Design review of the part built by this model. Coordinates are the model's own, in mm. Face numbers are marked on the shaded views. A direction names the side the tool comes from. Give positions to 0.01 mm unless a question says otherwise; leave off trailing zeros. Write each loop counter-clockwise with the first axis right and the second up, starting at its lowest first coordinate (ties: lowest second). Pieces come first, ordered by that corner, then holes. Notation, with made-up numbers: (35.25, -37) -> (91.25, -37) arc R7 cw to (91.25, -28) -> close; hole circle Ø7 at (-30, 0). An arc over 180 degrees is marked (long way). Write each question's results on one line, items separated by ' | '. Start each with the question number.
(1) Clearance check with flat-ended pins moving along their axes: pin 1 (1.1 mm diameter, centred on x = -34, y = -8, fed in from +Z); pin 2 (5 mm diameter, centred on x = 0.5, z = -31, fed in from +Y); pin 3 (5 mm diameter, centred on y = -5, z = -13.5, fed in from -X); pin 4 (2.5 mm diameter, centred on x = -0.15, y = -4.8, fed in from -Z). State where each tip first meets the part, or that it passes through.
(2) Take a section at B-B (z = -13). State the section outline as (x, y) points.
(3) Take a section at D-D (z = -30). State the section outline as (x, y) points, plus the area to 3 significant figures.
(4) Mouldability with a two-part tool opening along Y and no side actions: class the marked faces 1, 2 and 3 as released by +Y, released by -Y, zero draft, split by the parting line, or undercut.
(5) Take a section at C-C (z = -1.15). State the section outline as (x, y) points.
(6) Take a section at A-A (y = -2.5). State the section outline as (x, z) points, plus the area to 3 significant figures.
(7) To check wall thickness, follow probe 1 along Y at (x, z) = (-5.5, -12); probe 2 along X at (y, z) = (-15.9, -30); probe 3 along Z at (x, y) = (-1.5, 5). State the ranges of each line that lie inside material, in increasing order.
(8) For the marked faces 4, 5 and 6, list the 3-axis set-ups (+Z, -Z, +X, -X, +Y, -Y) from which the entire face can be reached by the end or side of a thin tool; tool diameter is ignored.
from build123d import *

# Parameters (mm, degrees)
ESBO_O3_W                 = 15
ESBO_O3_H                 = 34.8
RESSALTO_EXTRUS_O1_DEPTH  = 3
ESBO_O5_W                 = 15
ESBO_O5_H                 = 3
RESSALTO_EXTRUS_O2_DEPTH  = 18.6
ESBO_O6_W                 = 15
ESBO_O6_H                 = 3
RESSALTO_EXTRUS_O3_DEPTH  = 35
ESBO_O8_R                 = 1.5
CORTE_EXTRUS_O1_DEPTH     = 15
ESBO_O10_R                = 1.5
CORTE_EXTRUS_O3_DEPTH     = 15
CHANFRO2_SIZE             = 1.6
RESSALTO_EXTRUS_O5_DEPTH  = 15
ESBO_O14_R                = 1.5
RESSALTO_EXTRUS_O7_DEPTH  = 3
RESSALTO_EXTRUS_O9_DEPTH  = 26.8
CHANFRO6_SIZE             = 1
CHANFRO7_SIZE             = 1
CHANFRO8_SIZE             = 1
ESBO_O19_W                = 4.68
ESBO_O19_H                = 19.93
ESBO_O19_R                = 1.5
RESSALTO_EXTRUS_O10_DEPTH = 2
ESBO_O17_R                = 1.5
CORTE_EXTRUS_O4_DEPTH     = 7
CHANFRO4_SIZE             = 1
CHANFRO10_SIZE            = 1.6
CHANFRO11_SIZE            = 0.5


with BuildPart() as part:
    # Esboço3 → Ressalto-extrusão1 (new body)
    with BuildSketch(Plane.XY):
        with Locations((-2.101786792, 0.972895567)):
            Rectangle(ESBO_O3_W, ESBO_O3_H)
    extrude(amount=RESSALTO_EXTRUS_O1_DEPTH)

    # Esboço5 → Ressalto-extrusão2 (add)
    with BuildSketch(Plane(origin=(0, 0, 0), x_dir=(-1, 0, 0), z_dir=(0, 0, -1))):
        with Locations((2.101786792, 16.872895567)):
            Rectangle(ESBO_O5_W, ESBO_O5_H)
    extrude(amount=RESSALTO_EXTRUS_O2_DEPTH)

    # Esboço6 → Ressalto-extrusão3 (add)
    with BuildSketch(Plane(origin=(0, 0, 0), x_dir=(-1, 0, 0), z_dir=(0, 0, -1))):
        with Locations((2.101786792, -14.927104433)):
            Rectangle(ESBO_O6_W, ESBO_O6_H)
    extrude(amount=RESSALTO_EXTRUS_O3_DEPTH)

    # Esboço8 → Corte-extrusão1 (cut)
    with BuildSketch(Plane(origin=(0, 0, 0), x_dir=(-1, 0, 0), z_dir=(0, 0, -1))):
        with Locations((0.151786792, 12.802895567)):
            Circle(ESBO_O8_R)
        with Locations((0.151786792, -4.797104433)):
            Circle(ESBO_O8_R)
    extrude(amount=-CORTE_EXTRUS_O1_DEPTH, mode=Mode.SUBTRACT)

    # Esboço10 → Corte-extrusão3 (cut)
    with BuildSketch(Plane(origin=(0, -13.427104433, 0), x_dir=(1, 0, 0), z_dir=(0, 1, 0))):
        with Locations(Location((-2.101786792, 30, 0), (0, 0, 270))):
            Circle(ESBO_O10_R)
    extrude(amount=-CORTE_EXTRUS_O3_DEPTH, mode=Mode.SUBTRACT)

    # Chanfro2
    chanfro2_edges = [part.edges().sort_by_distance(p)[0] for p in [
        (-2.101786792, -13.427104433, -31.5),
    ]]
    chamfer(chanfro2_edges, length=CHANFRO2_SIZE)

    # Esboço11 → Ressalto-extrusão5 (add)
    with BuildSketch(Plane(origin=(5.398213208, 0, 0), x_dir=(0, 0, -1), z_dir=(1, 0, 0))):
        Polygon((7e-08, -7.367104433), (20, -7.367104433), (26.06, -13.427104433), (21.81735926, -13.427104379), (18.757359313, -10.367104433), (3.2e-08, -10.367104433), align=None)
    extrude(amount=-RESSALTO_EXTRUS_O5_DEPTH)

    # Esboço14 → Ressalto-extrusão7 (add)
    with BuildSketch(Plane.XY.offset(-7.35)):
        Polygon((-31.721786792, 6.502895567), (-31.721786792, -7.367104433), (-9.601786792, -7.367104433), (-9.601786792, -16.427104433), (-31.721786792, -16.427104433), (-36.401786792, -16.427104433), (-36.401786792, 6.502895567), align=None)
        with Locations((-34.001786792, 4.002895567)):
            Circle(ESBO_O14_R, mode=Mode.SUBTRACT)
    extrude(amount=RESSALTO_EXTRUS_O7_DEPTH)

    # Esboço16 → Ressalto-extrusão9 (add)
    with BuildSketch(Plane.ZY.offset(9.601786792)):
        Polygon((0, -13.427104433), (-4.35, -13.427104433), (-4.35, -16.427104433), (3, -16.427104433), (3, -13.427104433), align=None)
    extrude(amount=RESSALTO_EXTRUS_O9_DEPTH)

    # Chanfro6
    chanfro6_edges = [part.edges().sort_by_distance(p)[0] for p in [
        (-9.601786792, -11.897104433, -4.35),
        (-9.601786792, -11.897104433, -7.35),
    ]]
    chamfer(chanfro6_edges, length=CHANFRO6_SIZE)

    # Chanfro7
    chanfro7_edges = [part.edges().sort_by_distance(p)[0] for p in [
        (-9.601786792, -13.427104433, -14.58367963),
    ]]
    chamfer(chanfro7_edges, length=CHANFRO7_SIZE)

    # Chanfro8
    chanfro8_edges = [part.edges().sort_by_distance(p)[0] for p in [
        (-9.601786792, -13.427104433, -7.35),
    ]]
    chamfer(chanfro8_edges, length=CHANFRO8_SIZE)

    # Esboço19 → Ressalto-extrusão10 (add)
    with BuildSketch(Plane.XY.offset(-4.35)):
        with Locations((-34.061786792, -3.462104433)):
            Rectangle(ESBO_O19_W, ESBO_O19_H)
        with Locations((-34.001786792, 4.002895567)):
            Circle(ESBO_O19_R, mode=Mode.SUBTRACT)
    extrude(amount=RESSALTO_EXTRUS_O10_DEPTH)

    # Esboço17 → Corte-extrusão4 (cut)
    with BuildSketch(Plane(origin=(0, -13.427104433, 0), x_dir=(1, 0, 0), z_dir=(0, 1, 0))):
        with Locations(Location((-23.001786792, 1.15, 0), (0, 0, 270))):
            Circle(ESBO_O17_R)
    extrude(amount=-CORTE_EXTRUS_O4_DEPTH, mode=Mode.SUBTRACT)

    # Chanfro4
    chanfro4_edges = [part.edges().sort_by_distance(p)[0] for p in [
        (-23.001786792, -13.427104433, 3),
        (-36.401786792, -14.927104433, 3),
        (-2.101786792, 18.372895567, 3),
        (-9.601786792, 2.472895567, 3),
        (5.398213208, 16.872895567, -18.6),
        (-9.601786792, 16.872895567, -18.6),
        (-2.101786792, 18.372895567, -18.6),
        (-36.401786792, -13.427104433, 0.325),
        (5.398213208, -11.897104433, 0),
        (5.398213208, -13.427104433, -30.53),
        (-9.601786792, -13.427104433, -30.53),
        (5.398213208, -14.927104433, -35),
        (-9.601786792, -14.927104433, -35),
        (-2.101786792, -13.427104433, -35),
        (5.398213208, -13.427104433, -10.90867963),
        (-9.601786792, -11.897104433, 0),
        (5.398213208, -10.397104433, -23.03),
        (-9.601786792, -12.397104433, -20.787359313),
        (-9.601786792, -10.367104433, -2.175000016),
        (-9.601786792, -10.397104433, -23.03),
        (5.398213208, -10.367104433, -9.378679672),
        (5.398213208, -11.897104406, -20.287359286),
        (-9.601786792, 18.372895567, -7.8),
        (5.398213208, 18.372895567, -7.8),
        (-9.601786792, -10.367104433, -13.053679656),
        (5.398213208, 0.972895567, 3),
        (-20.661786792, -7.367104433, -4.35),
        (-20.661786792, -7.367104433, -7.35),
        (-31.721786792, 6.502895567, -4.85),
        (-36.401786792, 6.502895567, -4.85),
    ]]
    chamfer(chanfro4_edges, length=CHANFRO4_SIZE - 0.0001)  # a hair under: the kernel refuses the full size

    # Chanfro10
    chanfro10_edges = [part.edges().sort_by_distance(p)[0] for p in [
        (-23.001786792, -13.427104433, -2.65),
    ]]
    chamfer(chanfro10_edges, length=CHANFRO10_SIZE)

    # Chanfro11
    chanfro11_edges = [part.edges().sort_by_distance(p)[0] for p in [
        (-31.721786792, -3.962054433, -2.35),
        (-36.401786792, -5.462054433, -7.35),
        (-36.401786792, -4.462004433, -2.35),
        (-34.061786792, 6.502895567, -7.35),
        (-32.221736792, 6.002945567, -7.35),
        (-35.901836792, 6.002945567, -7.35),
        (-34.061786792, 6.502895567, -2.35),
        (-32.221736792, 6.002945567, -2.35),
        (-35.901836792, 6.002945567, -2.35),
        (-31.721786792, -1.432004433, -7.35),
    ]]
    chamfer(chanfro11_edges, length=CHANFRO11_SIZE)


solid = part.part
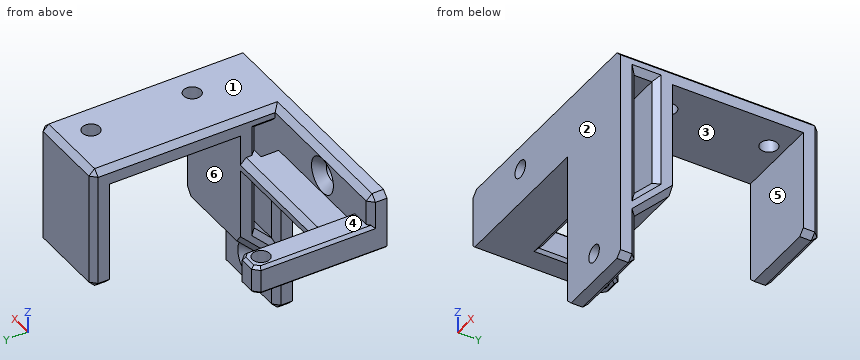
Report:
1) pin 1: z = -2.35 | pin 2: y = -13.43 | pin 3: x = -9.6 | pin 4: through
2) outline: (-9.6, -16.43) -> (5.4, -16.43) -> (5.4, -14.43) -> (4.4, -13.43) -> (-8.6, -13.43) -> (-9.6, -14.43) -> close; (-9.6, -9.37) -> (-8.6, -10.37) -> (4.4, -10.37) -> (5.4, -9.37) -> (5.4, -7.37) -> (-9.6, -7.37) -> close; (-9.6, 15.37) -> (5.4, 15.37) -> (5.4, 17.37) -> (4.4, 18.37) -> (-8.6, 18.37) -> (-9.6, 17.37) -> close
3) outline: (-9.6, -16.43) -> (-3.6, -16.43) -> (-3.6, -15.03) -> (-5.2, -13.43) -> (-8.6, -13.43) -> (-9.6, -14.43) -> close; (-0.6, -16.43) -> (5.4, -16.43) -> (5.4, -14.43) -> (4.4, -13.43) -> (1, -13.43) -> (-0.6, -15.03) -> close | area: 32.4 mm2
4) face 1: zero draft | face 2: released by -Y | face 3: undercut
5) outline: (-36.4, -16.43) -> (-24.5, -16.43) -> (-24.5, -15.03) -> (-26.1, -13.43) -> (-35.4, -13.43) -> (-36.4, -14.43) -> close; (-21.5, -16.43) -> (5.4, -16.43) -> (5.4, -14.43) -> (4.4, -13.43) -> (-19.9, -13.43) -> (-21.5, -15.03) -> close; (-9.6, -9.37) -> (-8.6, -10.37) -> (4.4, -10.37) -> (5.4, -9.37) -> (5.4, -7.37) -> (-9.6, -7.37) -> close; (-9.6, 15.37) -> (5.4, 15.37) -> (5.4, 17.37) -> (4.4, 18.37) -> (-8.6, 18.37) -> (-9.6, 17.37) -> close
6) outline: (-36.4, -6.85) -> (-35.9, -7.35) -> (-32.22, -7.35) -> (-31.72, -6.85) -> (-31.72, -2.85) -> (-32.22, -2.35) -> (-35.9, -2.35) -> (-36.4, -2.85) -> close; (-9.6, 0) -> (5.4, 0) -> (5.4, 2) -> (4.4, 3) -> (-8.6, 3) -> (-9.6, 2) -> close | area: 66.9 mm2
7) probe 1: -16.43 to -13.43, -10.37 to -7.37, 15.37 to 18.37 | probe 2: -9.6 to -3.6, -0.6 to 5.4 | probe 3: 0 to 3
8) face 4: +Z, -X, +Y | face 5: -Z, +X, -X | face 6: -Z, +X
